Read the model definition and answer for the solid it produces. Units are mm, in the model's axes. A direction names the side the tool comes from. Round coordinates to 2 decimals unless told otherwise and drop trailing zeros. Write each loop counter-clockwise with the first axis right and the second up, starting at its lowest first coordinate (ties: lowest second). Pieces come first, ordered by that corner, then holes. Notation, with made-up numbers: M -15.5,-34 L 11.5,-34 A23 ccw 11.5,-21 Z; hole C 12.25,37.5 d9. An arc over 180 degrees is marked long. Use one line per item in the form item = value. Start each with the question number.
```python
from build123d import *

# Parameters (mm, degrees)
BOSS_EXTRUDE1_DEPTH = 5
SKETCH1_R           = 1.6
CUT_EXTRUDE2_DEPTH  = 130.248833264


with BuildPart() as part:
    # Model → Boss-Extrude1 (new body)
    with BuildSketch(Plane.XY):
        Polygon((-12.44, -124.95), (-12.43, -124.94), (-12.42, -124.92), (-12.41, -124.91), (-12.4, -124.89), (-12.4, -119.97), (12.4, -119.97), (12.4, -124.89), (12.42, -124.93), (12.43, -124.94), (12.45, -124.95), (12.46, -124.96), (12.48, -124.97), (32.52, -124.97), (32.56, -124.95), (32.57, -124.94), (32.58, -124.92), (32.59, -124.91), (32.6, -124.89), (32.6, -112.48), (32.58, -112.44), (32.57, -112.43), (32.55, -112.42), (32.54, -112.41), (32.52, -112.4), (27.6, -112.4), (27.6, -87.6), (32.52, -87.6), (32.56, -87.58), (32.57, -87.57), (32.58, -87.55), (32.59, -87.54), (32.6, -87.52), (32.6, -62.48), (32.58, -62.44), (32.57, -62.43), (32.55, -62.42), (32.54, -62.41), (32.52, -62.4), (27.6, -62.4), (27.6, -37.6), (32.52, -37.6), (32.56, -37.58), (32.57, -37.57), (32.58, -37.55), (32.59, -37.54), (32.6, -37.52), (32.6, -12.48), (32.58, -12.44), (32.57, -12.43), (32.55, -12.42), (32.54, -12.41), (32.52, -12.4), (27.6, -12.4), (27.6, 12.4), (32.52, 12.4), (32.56, 12.42), (32.57, 12.43), (32.58, 12.45), (32.59, 12.46), (32.6, 12.48), (32.6, 37.52), (32.58, 37.56), (32.57, 37.57), (32.55, 37.58), (32.54, 37.59), (32.52, 37.6), (27.6, 37.6), (27.6, 62.4), (32.52, 62.4), (32.56, 62.42), (32.57, 62.43), (32.58, 62.45), (32.59, 62.46), (32.6, 62.48), (32.6, 87.52), (32.58, 87.56), (32.57, 87.57), (32.55, 87.58), (32.54, 87.59), (32.52, 87.6), (27.6, 87.6), (27.6, 112.4), (32.52, 112.4), (32.56, 112.42), (32.57, 112.43), (32.58, 112.45), (32.59, 112.46), (32.6, 112.48), (32.6, 124.89), (32.58, 124.93), (32.57, 124.94), (32.55, 124.95), (32.54, 124.96), (32.52, 124.97), (12.48, 124.97), (12.44, 124.95), (12.43, 124.94), (12.42, 124.92), (12.41, 124.91), (12.4, 124.89), (12.4, 119.97), (-12.4, 119.97), (-12.4, 124.89), (-12.42, 124.93), (-12.43, 124.94), (-12.45, 124.95), (-12.46, 124.96), (-12.48, 124.97), (-32.52, 124.97), (-32.56, 124.95), (-32.57, 124.94), (-32.58, 124.92), (-32.59, 124.91), (-32.6, 124.89), (-32.6, 112.48), (-32.58, 112.44), (-32.57, 112.43), (-32.55, 112.42), (-32.54, 112.41), (-32.52, 112.4), (-27.6, 112.4), (-27.6, 87.6), (-32.52, 87.6), (-32.56, 87.58), (-32.57, 87.57), (-32.58, 87.55), (-32.59, 87.54), (-32.6, 87.52), (-32.6, 62.48), (-32.58, 62.44), (-32.57, 62.43), (-32.55, 62.42), (-32.54, 62.41), (-32.52, 62.4), (-27.6, 62.4), (-27.6, 37.6), (-32.52, 37.6), (-32.56, 37.58), (-32.57, 37.57), (-32.58, 37.55), (-32.59, 37.54), (-32.6, 37.52), (-32.6, 12.48), (-32.58, 12.44), (-32.57, 12.43), (-32.55, 12.42), (-32.54, 12.41), (-32.52, 12.4), (-27.6, 12.4), (-27.6, -12.4), (-32.52, -12.4), (-32.56, -12.42), (-32.57, -12.43), (-32.58, -12.45), (-32.59, -12.46), (-32.6, -12.48), (-32.6, -37.52), (-32.58, -37.56), (-32.57, -37.57), (-32.55, -37.58), (-32.54, -37.59), (-32.52, -37.6), (-27.6, -37.6), (-27.6, -62.4), (-32.52, -62.4), (-32.56, -62.42), (-32.57, -62.43), (-32.58, -62.45), (-32.59, -62.46), (-32.6, -62.48), (-32.6, -87.52), (-32.58, -87.56), (-32.57, -87.57), (-32.55, -87.58), (-32.54, -87.59), (-32.52, -87.6), (-27.6, -87.6), (-27.6, -112.4), (-32.52, -112.4), (-32.56, -112.42), (-32.57, -112.43), (-32.58, -112.45), (-32.59, -112.46), (-32.6, -112.48), (-32.6, -124.89), (-32.58, -124.93), (-32.57, -124.94), (-32.55, -124.95), (-32.54, -124.96), (-32.52, -124.97), (-12.48, -124.97), align=None)
    extrude(amount=BOSS_EXTRUDE1_DEPTH)

    # Sketch1 → Cut-Extrude2 (cut, through all)
    with BuildSketch(Plane.XY.offset(5)):
        with Locations((0, 74.935)):
            Circle(SKETCH1_R)
        with Locations(Location((0, -74.935, 0), (0, 0, 180))):
            Circle(SKETCH1_R)
    extrude(amount=-CUT_EXTRUDE2_DEPTH, mode=Mode.SUBTRACT)


solid = part.part
```
Q1. Find section C-C on z = 1.55. Count the separate pieces of the cut face and the enclosed holes in it, and give its area (3 significant figures).
Q2. Each of these flat-tipped pins is pushed along its axis until it touches: pin 1 Ø1.5 at (y, z) = (-6.5, 2.5) entering from -X; pin 2 Ø5 at (x, y) = (0, -74.935) entering from +Z; pin 3 Ø2 at (x, z) = (-8, 1.5) entering from +Y. Where does it stop, or does it pass through?
Q3. A tool of negligible diameter and unlimited length cuts with its end or side. For faces 1 (the face through (-27.6, 50, 2)), 2 (the face through (-12.4, -122, 2)), 3 (the face through (30, 87.6, 2)), 4 (the face through (0, 119.97, 2)), from which of +Z, -Z, +X, -X, +Y, -Y can it reach the whole face along a straight path? Write none if from no direction.
Q4. Find section A-A on y = -10. Write down the section's boundary in (x, z), and give its area (3 significant figures).
Q5. For a pull along X with two mould halves and no side action, classify faces 5 (the face through (-30, 62.4, 2)), 6 (the face through (12.4, -122, 2)), 7 (the face through (-32.6, -75, 2)) as +X half, -X half, draft (parallel to the pull), parting line (faces both ways), or undercut.
Q6. Find section B-B on x = -6.5. Write down the section's boundary in (y, z).
Q7. Straight lines are drawn through the part: line 1 (Y direction, x = 0, z = 1.55) (3 decimals); line 2 (Y direction, x = 29, z = 4.6); line 3 (X direction, y = -75, z = 4.3). For each, find the intervals that lie inside material, in ascending order. Write a range as [from, to].
Response:
q1.separate_pieces = 1
q1.enclosed_holes = 2
q1.area = 14,800 mm²
q2.pin_1 = -27.6
q2.pin_2 = 5
q2.pin_3 = 119.97
q3.face_1 = +Z, -Z, -X
q3.face_2 = +Z, -Z, -Y
q3.face_3 = +Z, -Z, +X
q3.face_4 = +Z, -Z, +Y
q4.outline = M -27.6,0 L 27.6,0 L 27.6,5 L -27.6,5 Z
q4.area = 276 mm²
q5.face_5 = draft
q5.face_6 = undercut
q5.face_7 = -X half
q6.outline = M -119.97,0 L 119.97,0 L 119.97,5 L -119.97,5 Z
q7.line_1 = [-119.97, -76.535], [-73.335, 73.335], [76.535, 119.97]
q7.line_2 = [-124.97, -112.4], [-87.6, -62.4], [-37.6, -12.4], [12.4, 37.6], [62.4, 87.6], [112.4, 124.97]
q7.line_3 = [-32.6, -1.6], [1.6, 32.6]
